Read the model definition and answer for the solid it produces. Units are mm, in the model's axes. Coordinates: 2 decimals unless noted, no trailing zeros. Order: outer loops, then holes, each group sorted by start corner. A loop starts at its lowest first (then second) coordinate and runs counter-clockwise, first axis right, second up. Notation, with made-up numbers: M 37,44.5 L 60,44.5 A32 ccw 60,75.5 Z; hole C -0.5,-9.75 d8. An arc over 180 degrees is marked long. One line per question, with ' | ' between items. Start each with the question number.
1) Consider probe 1 along Y at (x, z) = (234.95, 7.25) (1 decimal); probe 2 along Y at (x, z) = (0, 5.75) (1 decimal); probe 3 along Y at (x, z) = (258.5, 15) (1 decimal). Determine where each line is inside the solid, lowest interval first.
2) Find section A-A, the plane x = -21.5. Write down the section's boundary in (y, z) (3 decimals).
3) Given P1, Ø1.5, axis at x = -17, y = 89.5, coming from the -Z side; P2, Ø9, axis at x = -261.874, y = 0, coming from the -Z side; P3, Ø6.5, axis at y = 0, z = 9.525, coming from the -X side; P4, Ø6.5, axis at y = 0, z = 9.525, coming from the +X side, each flat-ended and moving along its own axis, determine where each tip first touches the part or whether it passes through.
from build123d import *

# Parameters (mm, degrees)
F1_DEPTH  = 19.05
F3_D      = 15.0114
F3_DEPTH  = 14.224
F3_TIP    = 4.5098795482
F5_D      = 8.001
F5_DEPTH  = 25.4
F5_TIP    = 2.4037429064
F7_D      = 8.001
F7_DEPTH  = 25.4
F7_TIP    = 2.4037429064
F9_D      = 8.001
F9_DEPTH  = 14.224
F9_TIP    = 2.4037429064
F11_D     = 15.0114
F11_DEPTH = 14.224
F11_TIP   = 4.5098795482


# Not quite as in the source:
# - a feature names something its author has since deleted; it is built from what else it names


with BuildPart() as f1:
    # F0 (on Top) → F1 (new body)
    with BuildSketch(Plane.XY):
        Polygon((285.75, -295.275), (285.75, 295.275), (0, 295.275), (-285.75, 295.275), (-285.75, -295.275), align=None)
        with BuildLine():
            ThreePointArc((30.1625, 219.075), (-21.3281082875, 197.7468917125), (0, 249.2375))
            ThreePointArc((0, 249.2375), (21.3281082875, 240.4031082875), (30.1625, 219.075))
        make_face(mode=Mode.SUBTRACT)
    extrude(amount=F1_DEPTH)

    # F3
    with Locations(Plane(origin=(0, 0, 0), x_dir=(1, 0, 0), z_dir=(0, 0, -1))):
        with Locations((-261.874, 244.475), (261.874, 244.475), (-261.874, 0), (261.874, 0), (261.874, -244.475), (-261.874, -244.475)):
            Hole(F3_D / 2, depth=F3_DEPTH)
            with Locations((0, 0, -(F3_DEPTH + F3_TIP / 2))):  # 118° drill point
                Cone(0, F3_D / 2, F3_TIP, mode=Mode.SUBTRACT)

    # F5
    with Locations(Plane.YZ.offset(285.75)):
        with Locations((-244.475, 9.525), (0, 9.525), (233.3625, 9.525)):
            Hole(F5_D / 2, depth=F5_DEPTH)
            with Locations((0, 0, -(F5_DEPTH + F5_TIP / 2))):  # 118° drill point
                Cone(0, F5_D / 2, F5_TIP, mode=Mode.SUBTRACT)

    # F7
    with Locations(Plane(origin=(-285.75, 0, 0), x_dir=(0, -1, 0), z_dir=(-1, 0, 0))):
        with Locations((0, 9.525), (244.475, 9.525), (-244.475, 9.525)):
            Hole(F7_D / 2, depth=F7_DEPTH)
            with Locations((0, 0, -(F7_DEPTH + F7_TIP / 2))):  # 118° drill point
                Cone(0, F7_D / 2, F7_TIP, mode=Mode.SUBTRACT)

    # F9
    with Locations(Plane(origin=(0, 0, 0), x_dir=(1, 0, 0), z_dir=(0, 0, -1))):
        with Locations((-234.95, 279.4), (0, 279.4), (234.95, 279.4)):
            Hole(F9_D / 2, depth=F9_DEPTH)
            with Locations((0, 0, -(F9_DEPTH + F9_TIP / 2))):  # 118° drill point
                Cone(0, F9_D / 2, F9_TIP, mode=Mode.SUBTRACT)

    # F11
    with Locations(Plane(origin=(0, 0, 0), x_dir=(1, 0, 0), z_dir=(0, 0, -1))):
        with Locations((-234.95, -271.399), (234.95, -271.399)):
            Hole(F11_D / 2, depth=F11_DEPTH)
            with Locations((0, 0, -(F11_DEPTH + F11_TIP / 2))):  # 118° drill point
                Cone(0, F11_D / 2, F11_TIP, mode=Mode.SUBTRACT)


solid = f1.part
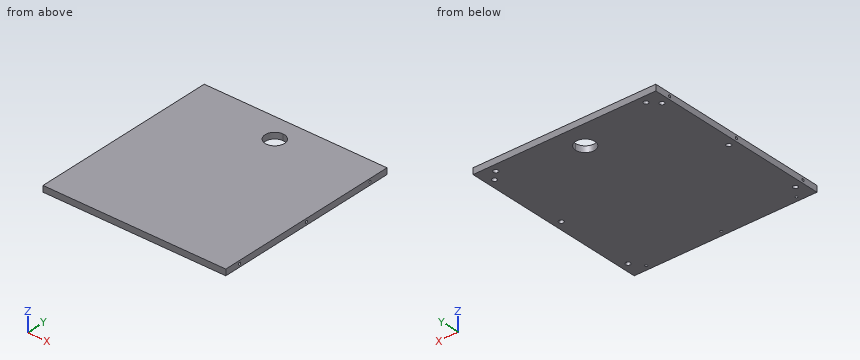
Report:
1) probe 1: y = -295.3 to -283.4, -275.4 to 263.9, 278.9 to 295.3 | probe 2: y = -295.3 to -283.4, -275.4 to 188.9, 249.2 to 295.3 | probe 3: y = -295.3 to -249.7, -239.3 to -5.2, 5.2 to 239.3, 249.7 to 295.3
2) outline: M -295.275,0 L 197.92,0 L 197.92,19.05 L -295.275,19.05 Z; M 240.23,0 L 295.275,0 L 295.275,19.05 L 240.23,19.05 Z
3) P1: stops at z = 0 | P2: stops at z = 16.03 | P3: stops at x = -255.11 | P4: stops at x = 255.11
